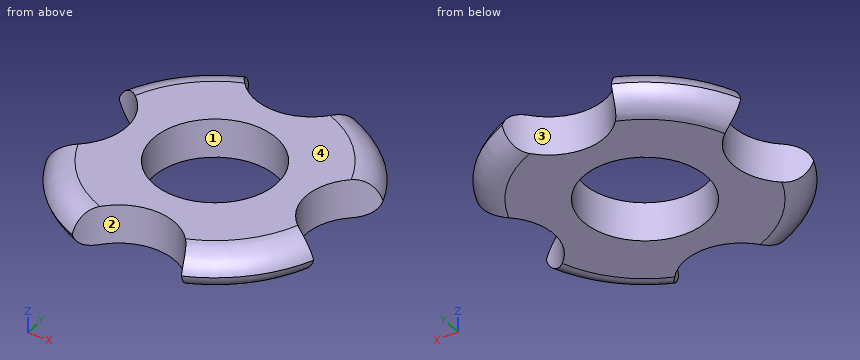
from build123d import *

# Parameters (mm, degrees)
F0_R         = 26.25
F1_DEPTH     = 7
F2_R         = 11.125
F3_DEPTH     = 25.4
F4_R         = 10.16
F4_R_2       = 9.6723514766
F5_DEPTH     = 25.4
F6_T2_ANGLE  = 101.8963155292
F6_T4_ANGLE  = 100.8121389037
F6_T6_ANGLE  = 100.8121389037
F6_T8_ANGLE  = 100.8121389037
F6_T10_ANGLE = 100.8121389037
F6_T12_ANGLE = 101.8963155292
F6_T14_ANGLE = 101.8963155292
F6_T16_ANGLE = 101.8963155292


# Not quite as in the source:
# - a fillet or chamfer that OpenCascade refuses, or shapes differently, is made with other operations: its cross-section is extruded or revolved along the edge and cut away or added


with BuildPart() as f1:
    # F0 (on Top) → F1 (new body)
    with BuildSketch(Plane.XY):
        Circle(F0_R)
    extrude(amount=F1_DEPTH)

    # F2 (on face) → F3 (cut)
    with BuildSketch(Plane.XY.offset(7)):
        Circle(F2_R)
    extrude(amount=-F3_DEPTH, mode=Mode.SUBTRACT)

    # F4 (on face) → F5 (cut)
    with BuildSketch(Plane.XY.offset(7)):
        with Locations((0, -26.25)):
            Circle(F4_R)
        with Locations((-26.25, 0)):
            Circle(F4_R)
        with Locations((0, 26.25)):
            Circle(F4_R)
        with Locations((26.25, 0)):
            Circle(F4_R_2)
    extrude(amount=-F5_DEPTH, mode=Mode.SUBTRACT)

    # F6: fillet of radius 5.08 on 8 edges, made by hand

    # F6_s1 → F6_t2 (revolve, cut)
    with BuildSketch(Plane(origin=(0, 0, 0), x_dir=(0, 0, 1), z_dir=(-0.995551765, 0.0942161515, 0))):
        with BuildLine():
            ThreePointArc((5.08, -26.25), (1.4878975516, -24.7621024484), (0, -21.17))
            Line((0, -21.17), (0, -26.25))
            Line((0, -26.25), (5.08, -26.25))
        make_face()
    revolve(axis=Axis((0, 0, 0), (0, 0, 1)), revolution_arc=F6_T2_ANGLE, mode=Mode.SUBTRACT)

    # F6_s3 → F6_t4 (revolve, cut)
    with BuildSketch(Plane(origin=(0, 0, 0), x_dir=(0, 0, 1), z_dir=(0.0942137746, 0.9955519899, 0))):
        with BuildLine():
            ThreePointArc((5.08, -26.25), (1.4878975516, -24.7621024484), (0, -21.17))
            Line((0, -21.17), (0, -26.25))
            Line((0, -26.25), (5.08, -26.25))
        make_face()
    revolve(axis=Axis((0, 0, 0), (0, 0, 1)), revolution_arc=F6_T4_ANGLE, mode=Mode.SUBTRACT)

    # F6_s5 → F6_t6 (revolve, cut)
    with BuildSketch(Plane(origin=(0, 0, 0), x_dir=(0, 0, 1), z_dir=(0.9955519899, -0.0942137746, 0))):
        with BuildLine():
            ThreePointArc((5.08, -26.25), (1.4878975516, -24.7621024484), (0, -21.17))
            Line((0, -21.17), (0, -26.25))
            Line((0, -26.25), (5.08, -26.25))
        make_face()
    revolve(axis=Axis((0, 0, 0), (0, 0, 1)), revolution_arc=F6_T6_ANGLE, mode=Mode.SUBTRACT)

    # F6_s7 → F6_t8 (revolve, cut)
    with BuildSketch(Plane(origin=(0, 0, 0), x_dir=(0, 0, 1), z_dir=(0.9955519899, -0.0942137746, 0))):
        with BuildLine():
            ThreePointArc((1.92, -26.25), (5.5121024484, -24.7621024484), (7, -21.17))
            Line((7, -21.17), (7, -26.25))
            Line((7, -26.25), (1.92, -26.25))
        make_face()
    revolve(axis=Axis((0, 0, 7), (0, 0, 1)), revolution_arc=F6_T8_ANGLE, mode=Mode.SUBTRACT)

    # F6_s9 → F6_t10 (revolve, cut)
    with BuildSketch(Plane(origin=(0, 0, 0), x_dir=(0, 0, 1), z_dir=(0.0942137746, 0.9955519899, 0))):
        with BuildLine():
            ThreePointArc((1.92, -26.25), (5.5121024484, -24.7621024484), (7, -21.17))
            Line((7, -21.17), (7, -26.25))
            Line((7, -26.25), (1.92, -26.25))
        make_face()
    revolve(axis=Axis((0, 0, 7), (0, 0, 1)), revolution_arc=F6_T10_ANGLE, mode=Mode.SUBTRACT)

    # F6_s11 → F6_t12 (revolve, cut)
    with BuildSketch(Plane(origin=(0, 0, 0), x_dir=(0, 0, 1), z_dir=(-0.995551765, 0.0942161515, 0))):
        with BuildLine():
            ThreePointArc((1.92, -26.25), (5.5121024484, -24.7621024484), (7, -21.17))
            Line((7, -21.17), (7, -26.25))
            Line((7, -26.25), (1.92, -26.25))
        make_face()
    revolve(axis=Axis((0, 0, 7), (0, 0, 1)), revolution_arc=F6_T12_ANGLE, mode=Mode.SUBTRACT)

    # F6_s13 → F6_t14 (revolve, cut)
    with BuildSketch(Plane(origin=(0, 0, 0), x_dir=(0, 0, 1), z_dir=(-0.1130316961, -0.9935913826, 0))):
        with BuildLine():
            ThreePointArc((1.92, -26.25), (5.5121024484, -24.7621024484), (7, -21.17))
            Line((7, -21.17), (7, -26.25))
            Line((7, -26.25), (1.92, -26.25))
        make_face()
    revolve(axis=Axis((0, 0, 7), (0, 0, 1)), revolution_arc=F6_T14_ANGLE, mode=Mode.SUBTRACT)

    # F6_s15 → F6_t16 (revolve, cut)
    with BuildSketch(Plane(origin=(0, 0, 0), x_dir=(0, 0, 1), z_dir=(-0.1130316961, -0.9935913826, 0))):
        with BuildLine():
            ThreePointArc((5.08, -26.25), (1.4878975516, -24.7621024484), (0, -21.17))
            Line((0, -21.17), (0, -26.25))
            Line((0, -26.25), (5.08, -26.25))
        make_face()
    revolve(axis=Axis((0, 0, 0), (0, 0, 1)), revolution_arc=F6_T16_ANGLE, mode=Mode.SUBTRACT)


solid = f1.part
Geometry: final body of the model. Coordinates: model frame, mm. Face numbers are marked on the shaded views. Round coordinates to 2 decimals unless told otherwise and drop trailing zeros. Loops run counter-clockwise (first coordinate to the right, second up) from the corner with the lowest first, then second, coordinate; pieces in that order, holes last. Notation, with made-up numbers: M 4,-5.5 L 22,-5.5 A14 ccw 22,10.5 Z; hole C 10,17 d11. An arc over 180 degrees is marked long. Put each result on its own line as item: value. Start each with the question number.
(1) Section query D-D (z = 4.75). Return loops of the section in (x, y) (3 decimals), then the cut area to 3 significant figures.
(2) Section query C-C (z = 1.75). Return loops of the section in (x, y) (3 decimals), then the cut area to 3 significant figures.
(3) Contact query for flat-ended pins moving along their axis: pin 1 Ø3 at (x, z) = (-0.5, 3.5) entering from -Y; pin 2 Ø4 at (x, z) = (10, 0.5) entering from +Y; pin 3 Ø2 at (y, z) = (9, 4) entering from -X. Output: stop coordinate, or through.
(4) Material intervals for line 1 along Y through (x, z) = (-20, 3.25); line 2 along Y through (x, z) = (21, 5); line 3 along X through (y, z) = (-1, 3.5), sorted ascending. Write a range as [from, to].
(5) Draft query along Y for the marked faces 1, 2, 3 and 4. Return one class per face: +Y half, -Y half, draft (parallel to the pull), parting line (faces both ways), or undercut.
(6) Section query A-A (x = 0). Return loops of the section in (y, z) (3 decimals), then the cut area to 3 significant figures.
(7) Section query B-B (y = 0). Return loops of the section in (x, z) (3 decimals).
Findings below:
1. outline: M -23.437,-9.763 A25.389 ccw -9.763,-23.437 A10.16 cw 9.763,-23.437 A25.389 ccw 23.621,-9.308 A9.672 cw 23.621,9.308 A25.389 ccw 9.763,23.437 A10.16 cw -9.763,23.437 A25.389 ccw -23.437,9.763 A10.16 cw Z; hole C 0,0 d22.25
1. area: 1,120 mm2
2. outline: M -23.07,-9.649 A25.006 ccw -9.649,-23.07 A10.16 cw 9.649,-23.07 A25.006 ccw 23.254,-9.197 A9.672 cw 23.254,9.197 A25.006 ccw 9.649,23.07 A10.16 cw -9.649,23.07 A25.006 ccw -23.07,9.649 A10.16 cw Z; hole C 0,0 d22.25
2. area: 1,090 mm2
3. pin 1: stops at y = -16.29
3. pin 2: stops at y = 23.58
3. pin 3: stops at x = -24.01
4. line 1: y = [-16.47, -8.01], [8.01, 16.47]
4. line 2: y = [-13.95, -8.12], [8.12, 13.95]
4. line 3: x = [-16.14, -11.08], [11.08, 16.63]
5. face 1: undercut
5. face 2: -Y half
5. face 3: +Y half
5. face 4: draft
6. outline: M -16.09,0 L -11.125,0 L -11.125,7 L -16.09,7 Z; M 11.125,0 L 16.09,0 L 16.09,7 L 11.125,7 Z
6. area: 69.5 mm2
7. outline: M -16.09,0 L -11.125,0 L -11.125,7 L -16.09,7 Z; M 11.125,0 L 16.578,0 L 16.578,7 L 11.125,7 Z
